Can you work these out from the model? Positions are in its coordinate system, mm. Coordinates: 2 decimals unless noted, no trailing zeros. Order: outer loops, then holes, each group sorted by start corner. A loop starts at its lowest first (then second) coordinate and runs counter-clockwise, first axis right, second up. Notation, with made-up numbers: (-39.75, 9.5) - (-32.75, 9.5) arc R22 cw to (-32.75, 38.5) - close; hole circle Ø4 at (-28, 46.5). An arc over 180 degrees is marked (long way). Use a Markdown table: item, result. Add a question column.
(1) I want a section at A-A (x = -157). List the corners of the cut face in (y, z) for me, and give its area (3 significant figures).
(2) For pin 1 Ø1.5 at (x, z) = (-559.5, -15) entering from +Y; pin 2 Ø6 at (x, z) = (-658.5, -10.5) entering from -Y; pin 3 Ø4 at (x, z) = (-182.5, -11) entering from +Y, each with a flat end and sliding along its axis, tell me the tip position at first contact or that it passes through.
(3) If I drill on L1, parallel to X at y = -461.5, z = -8.75; L2, parallel to X at y = -1517.5, z = -8.5; L3, parallel to Y at x = -133.5, z = -21.5, over which ranges is the centre line in solid material (lowest first)? Write a range as [from, to].
(4) I want a section at C-C (z = -20.75). List the corners of the cut face in (x, y) for me.
(5) I want a section at B-B (y = -228). List the corners of the cut face in (x, z) for me, and give its area (3 significant figures).
```python
from build123d import *

# Parameters (mm, degrees)
EXTRUDE_THIN1_START = -26.269809
EXTRUDE_THIN1_DEPTH = 19


with BuildPart() as part:
    # Sketch2 → Extrude-Thin1 (new body)
    with BuildSketch(Plane(origin=(-2.158928767, 13.648417367, 0), x_dir=(1, 0, 0), z_dir=(0, 0, 1)).offset(EXTRUDE_THIN1_START)):
        with BuildLine():
            Line((-841.621500671, -1754.223207182), (-17.391917272, 8.133954365))
            ThreePointArc((-17.391917272, 8.133954365), (8.133954365, 17.391917272), (17.391917272, -8.133954365))
            Line((17.391917272, -8.133954365), (-806.837666127, -1770.491115912))
            ThreePointArc((-806.837666127, -1770.491115912), (-832.363537764, -1779.749078819), (-841.621500671, -1754.223207182))
        make_face()
        with BuildLine():
            Line((-837.998184572, -1755.917781008), (-13.768601173, 6.439380539))
            ThreePointArc((-13.768601173, 6.439380539), (6.439380539, 13.768601173), (13.768601173, -6.439380539))
            Line((13.768601173, -6.439380539), (-810.460982226, -1768.796542086))
            ThreePointArc((-810.460982226, -1768.796542086), (-830.668963938, -1776.12576272), (-837.998184572, -1755.917781008))
        make_face(mode=Mode.SUBTRACT)
    extrude(amount=EXTRUDE_THIN1_DEPTH)


solid = part.part
```
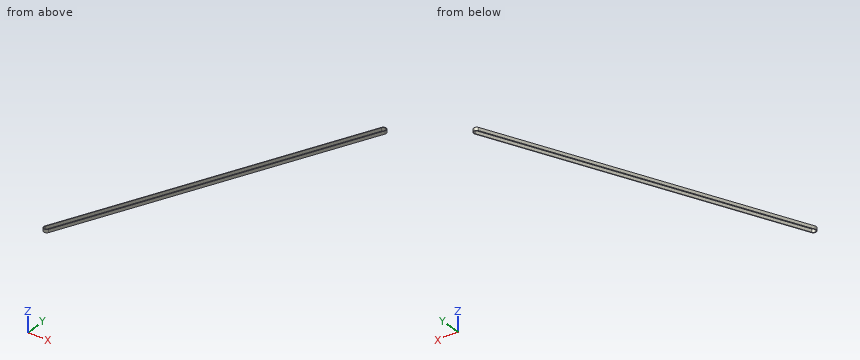
Answers follow:
| question | item | result |
|---|---|---|
| 1 | outline | (-362.75, -26.27) - (-353.31, -26.27) - (-353.31, -7.27) - (-362.75, -7.27) - close; (-281.55, -26.27) - (-272.11, -26.27) - (-272.11, -7.27) - (-281.55, -7.27) - close |
| 1 | area | 359 mm² |
| 2 | pin 1 | stops at y = -1131.13 |
| 2 | pin 2 | stops at y = -1441.47 |
| 2 | pin 3 | stops at y = -322.36 |
| 3 | L1 | x = [-245.58, -241.16], [-207.6, -203.18] |
| 3 | L2 | x = [-739.45, -735.04], [-701.48, -697.06] |
| 3 | L3 | y = [-312.5, -303.06], [-231.3, -221.86] |
| 4 | outline | (-843.78, -1740.57) arc R19.2 ccw to (-809, -1756.84) - (15.23, 5.51) arc R19.2 ccw to (-19.55, 21.78) - close; hole (-840.16, -1742.27) arc R15.2 ccw to (-812.62, -1755.15) - (11.61, 7.21) arc R15.2 ccw to (-15.93, 20.09) - close |
| 5 | outline | (-136.37, -26.27) - (-131.95, -26.27) - (-131.95, -7.27) - (-136.37, -7.27) - close; (-98.39, -26.27) - (-93.98, -26.27) - (-93.98, -7.27) - (-98.39, -7.27) - close |
| 5 | area | 168 mm² |
